```python
from build123d import *

# Parameters (mm, degrees)
F3_R = 15
F4_R = 5
F5_T = -1.25


with BuildPart() as f2:
    # F1 (on Front) → F2 (revolve)
    with BuildSketch(Plane.XZ):
        Polygon((-15, -20), (0, -20), (0, 20), (0, 60), (-10, 60), (-10, 37.5), (-15, 25), align=None)
    revolve(axis=Axis((0, 0, 0), (0, 0, -1)))

    # F3
    f3_edges = [f2.edges().sort_by_distance(p)[0] for p in [
        (15, 0, 25),
        (10, 0, 37.5),
    ]]
    fillet(f3_edges, radius=F3_R)

    # F4
    f4_edges = [f2.edges().sort_by_distance(p)[0] for p in [
        (15, 0, -20),
    ]]
    fillet(f4_edges, radius=F4_R)

    # F5
    f5_openings = [f2.faces().sort_by_distance(p)[0] for p in [
        (0, 0, 60),
    ]]
    offset(amount=F5_T, openings=f5_openings)


solid = f2.part
```
The listing builds one solid part. Answer for the finished solid, in the listing's coordinates (mm). A direction names the side the tool comes from. Give positions to 0.01 mm unless a question says otherwise; leave off trailing zeros. Order: outer loops, then holes, each group sorted by start corner. A loop starts at its lowest first (then second) coordinate and runs counter-clockwise, first axis right, second up.
Item 1: Given pin 1 Ø3 at (x, z) = (10, -4) entering from -Y; pin 2 Ø6 at (x, y) = (2, -1.5) entering from +Z; pin 3 Ø12 at (x, z) = (2.5, 34.5) entering from +Y, each flat-ended and moving along its own axis, determine where each tip first touches the part or whether it passes through.
From the geometry:
pin 1: stops at y = -12.36
pin 2: stops at z = -18.75
pin 3: stops at y = 13.49
Item 2: The part is cut by section B-B, the plane z = 13.5. Give the vertices of the cut face in (x, y).
From the geometry:
outline: circle Ø30 at (0, 0); hole circle Ø27.5 at (0, 0)
Item 3: The part is cut by section A-A, the plane z = 51. Give the vertices of the cut face in (x, y).
From the geometry:
outline: circle Ø20 at (0, 0); hole circle Ø17.5 at (0, 0)
Item 4: Which of the six approach directions +Z, -Z, +X, -X, +Y, -Y give full straight-line access (tool end or side, diameter ignored) to faces 5 (the face through (0, 0, -20)), 6 (the face through (-9.625, 3.031, 33.907)), 7 (the face through (-8.346, 2.628, 50.057))?
From the geometry:
face 5: -Z, +X, -X, +Y, -Y
face 6: none
face 7: +Z
Item 5: For a pull along Y with two mould halves and no side action, classify faces 1 (the face through (0, -9, 60)), 2 (the face through (0, 0, -18.75)), 3 (the face through (14.985, 0.66, 3.296)), 4 (the face through (2.981, -13.423, 3.296)) as pulls with the +Y half, pulls with the -Y half, needs draft (parallel to the pull), parting line crosses it, or undercut.
From the geometry:
face 1: needs draft
face 2: undercut
face 3: parting line crosses it
face 4: undercut
Item 6: Find the intervals of material crossed by probe 1 along X at (y, z) = (0, -4); probe 2 along X at (y, z) = (0, 52), in increasing order.
From the geometry:
probe 1: x = -15 to -13.75, 13.75 to 15
probe 2: x = -10 to -8.75, 8.75 to 10
